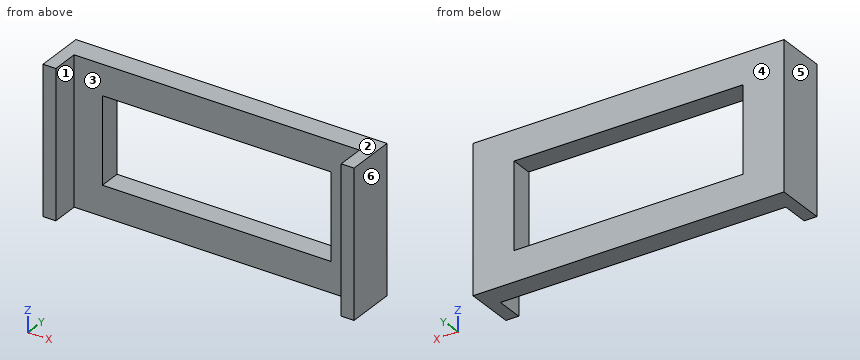
from build123d import *

# Parameters (mm, degrees)
F0_W     = 85
F0_H     = 40
F1_DEPTH = 6
F2_W     = 62.5
F2_H     = 23.5
F3_DEPTH = 25
F4_W     = 3.5
F4_H     = 40
F5_DEPTH = 7.5


with BuildPart() as f1:
    # F0 (on Front) → F1 (new body)
    with BuildSketch(Plane.XZ):
        Rectangle(F0_W, F0_H)
    extrude(amount=F1_DEPTH)

    # F2 (on face) → F3 (cut)
    with BuildSketch(Plane.XZ.offset(6)):
        Rectangle(F2_W, F2_H)
    extrude(amount=-F3_DEPTH, mode=Mode.SUBTRACT)

    # F4 (on face) → F5 (join)
    with BuildSketch(Plane.XZ.offset(6)):
        with Locations((40.75, 0)):
            Rectangle(F4_W, F4_H)
        with Locations((-40.75, 0)):
            Rectangle(F4_W, F4_H)
    extrude(amount=F5_DEPTH)


solid = f1.part
For this review, take the finished solid that the model builds, in its own axes (mm). Face numbers are marked on the shaded views. A direction names the side the tool comes from. Round coordinates to 2 decimals unless told otherwise and drop trailing zeros. Loops run counter-clockwise (first coordinate to the right, second up) from the corner with the lowest first, then second, coordinate; pieces in that order, holes last. Notation, with made-up numbers: (-17, 44.25) - (0, 44.25) arc R27 ccw to (0, 78.25) - close; hole circle Ø10 at (45, 34). An arc over 180 degrees is marked (long way). One line per item, written item: value. Start each with the question number.
Item 1: Take a section at A-A (z = -2.5). Give the boundary of the cut face in (x, y).
Item 2: Take a section at C-C (x = -16.5). Give the boundary of the cut face in (y, z), plus the area to 3 significant figures.
Item 3: Take a section at B-B (y = -3). Give the boundary of the cut face in (x, z), plus the area to 3 significant figures.
Item 4: For L1, parallel to X at y = -7.5, z = 10.5; L2, parallel to X at y = -3, z = -11; L3, parallel to Z at x = -2.5, y = -2, list the stretches that pass through material, from the lowest coordinate up.
Item 5: For the marked faces 1 and 2, list the 3-axis set-ups (+Z, -Z, +X, -X, +Y, -Y) from which the entire face can be reached by the end or side of a thin tool; tool diameter is ignored.
Item 6: Take a section at D-D (y = -12.25). Give the boundary of the cut face in (x, z), plus the area to 3 significant figures.
Item 7: Clearance check with flat-ended pins moving along their axes: pin 1 Ø5 at (x, z) = (27, 1) entering from -Y; pin 2 Ø12 at (x, z) = (17, -8.5) entering from -Y. State where each tip first meets the part, or that it passes through.
Item 8: The part is to be moulded in two halves that separate along X. For the marked faces 3, 4, 5 and 6, say which applies: +X half, -X half, draft (parallel to the pull), parting line (faces both ways), or undercut.
Answer below:
1. outline: (-42.5, -13.5) - (-39, -13.5) - (-39, -6) - (-31.25, -6) - (-31.25, 0) - (-42.5, 0) - close; (31.25, -6) - (39, -6) - (39, -13.5) - (42.5, -13.5) - (42.5, 0) - (31.25, 0) - close
2. outline: (-6, -20) - (0, -20) - (0, -11.75) - (-6, -11.75) - close; (-6, 11.75) - (0, 11.75) - (0, 20) - (-6, 20) - close
2. area: 99.0 mm2
3. outline: (-42.5, -20) - (42.5, -20) - (42.5, 20) - (-42.5, 20) - close; hole (-31.25, -11.75) - (31.25, -11.75) - (31.25, 11.75) - (-31.25, 11.75) - close
3. area: 1,930 mm2
4. L1: x = -42.5 to -39, 39 to 42.5
4. L2: x = -42.5 to -31.25, 31.25 to 42.5
4. L3: z = -20 to -11.75, 11.75 to 20
5. face 1: +Z, -Z, -Y
5. face 2: +Z, +X, -X, +Y, -Y
6. outline: (-42.5, -20) - (-39, -20) - (-39, 20) - (-42.5, 20) - close; (39, -20) - (42.5, -20) - (42.5, 20) - (39, 20) - close
6. area: 280 mm2
7. pin 1: passes through
7. pin 2: stops at y = -6
8. face 3: undercut
8. face 4: draft
8. face 5: -X half
8. face 6: +X half
